Work out the finished part from the listing and answer in its coordinate system (mm). A direction names the side the tool comes from. Coordinates: 2 decimals unless noted, no trailing zeros. Order: outer loops, then holes, each group sorted by start corner. A loop starts at its lowest first (then second) coordinate and runs counter-clockwise, first axis right, second up. Notation, with made-up numbers: (-14.75, 9.5) -> (13.25, 9.5) arc R25 ccw to (13.25, 38.5) -> close; hole circle Ø1 at (70.25, 55.5). An arc over 180 degrees is marked (long way). Use one line per item in the form item = value.
from build123d import *

# Parameters (mm, degrees)
BASE_FLANGE1_DEPTH           = 408.432
SKETCH2_W                    = 2.032
SKETCH2_H                    = 34.036
BOSS_EXTRUDE1_DEPTH          = 25.4
EDGE_FLANGE1_STRIP_W         = 14.478
EDGE_FLANGE1_STRIP_H         = 2.032
EDGE_FLANGE1_STRIP_CUT_DEPTH = 34.036
EDGE_FLANGE1_DEPTH           = 34.036
SKETCH6_R                    = 2.4511
CUT_EXTRUDE1_DEPTH           = 438.764339256
SKETCH7_R                    = 4.3688
CUT_EXTRUDE2_DEPTH           = 438.764339256
SKETCH8_R                    = 2.4511
CUT_EXTRUDE3_DEPTH           = 463.94863897
FILLET1_R                    = 3.175


# Sheet-metal steps are written as plain solids
with BuildPart() as part:
    # Sketch1 → Base-Flange1 (new body)
    with BuildSketch(Plane(origin=(0, 0, 0), x_dir=(0, 0, -1), z_dir=(1, 0, 0))):
        with BuildLine():
            Line((22.225, 0), (5.207, 0))
            ThreePointArc((5.207, 0), (1.52509499, 1.52509499), (0, 5.207))
            Line((0, 5.207), (0, 39.243))
            ThreePointArc((0, 39.243), (1.52509499, 42.92490501), (5.207, 44.45))
            Line((5.207, 44.45), (22.225, 44.45))
            Line((22.225, 44.45), (22.225, 42.418))
            Line((22.225, 42.418), (5.207, 42.418))
            ThreePointArc((5.207, 42.418), (2.96193597, 41.48806403), (2.032, 39.243))
            Line((2.032, 39.243), (2.032, 5.207))
            ThreePointArc((2.032, 5.207), (2.96193597, 2.96193597), (5.207, 2.032))
            Line((5.207, 2.032), (22.225, 2.032))
            Line((22.225, 2.032), (22.225, 0))
        make_face()
    extrude(amount=BASE_FLANGE1_DEPTH)

    # Sketch2 → Boss-Extrude1 (add)
    with BuildSketch(Plane(origin=(408.432, 0, 0), x_dir=(0, 0, -1), z_dir=(1, 0, 0))):
        with Locations((1.016, 22.225)):
            Rectangle(SKETCH2_W, SKETCH2_H)
    boss_extrude1 = extrude(amount=BOSS_EXTRUDE1_DEPTH)

    # Edge-Flange1 strip (across the edge) → Edge-Flange1 strip cut (cut)
    with BuildSketch(Plane(origin=(433.832, 39.243, -2.032), x_dir=(-1, 0, 0), z_dir=(0, -1, 0))):
        with Locations((-2.032, -1.016)):
            Rectangle(EDGE_FLANGE1_STRIP_W, EDGE_FLANGE1_STRIP_H)
    edge_flange1_strip_cut = extrude(amount=EDGE_FLANGE1_STRIP_CUT_DEPTH, mode=Mode.SUBTRACT)

    # Edge-Flange1 section (across the edge) → Edge-Flange1 (add)
    with BuildSketch(Plane(origin=(433.832, 39.243, -2.032), x_dir=(-1, 0, 0), z_dir=(0, -1, 0))):
        with BuildLine():
            Line((0, 3.175), (0, 36.068))
            Line((0, 36.068), (2.032, 36.068))
            Line((2.032, 36.068), (2.032, 3.175))
            ThreePointArc((2.032, 3.175), (2.96193597, 0.92993597), (5.207, 0))
            Line((5.207, 0), (5.207, -2.032))
            ThreePointArc((5.207, -2.032), (1.52509499, -0.50690501), (0, 3.175))
        make_face()
    edge_flange1 = extrude(amount=EDGE_FLANGE1_DEPTH)

    # Mirror1: Boss-Extrude1, Edge-Flange1 strip cut, Edge-Flange1 across plane
    add(boss_extrude1.mirror(Plane.ZY.offset(-204.216)))
    add(edge_flange1_strip_cut.mirror(Plane.ZY.offset(-204.216)), mode=Mode.SUBTRACT)
    add(edge_flange1.mirror(Plane.ZY.offset(-204.216)))

    # Sketch6 → Cut-Extrude1 (cut, through all)
    with BuildSketch(Plane(origin=(0, 44.45, 0), x_dir=(1, 0, 0), z_dir=(0, 1, 0))):
        with Locations(Location((25.4, 15.875, 0), (0, 0, 270))):
            Circle(SKETCH6_R)
        with Locations(Location((383.032, 15.875, 0), (0, 0, 270))):
            Circle(SKETCH6_R)
    extrude(amount=-CUT_EXTRUDE1_DEPTH, mode=Mode.SUBTRACT)

    # Sketch7 → Cut-Extrude2 (cut, through all)
    with BuildSketch(Plane.XY):
        with Locations((50.8, 22.225)):
            Circle(SKETCH7_R)
        with Locations((357.632, 22.225)):
            Circle(SKETCH7_R)
    extrude(amount=-CUT_EXTRUDE2_DEPTH, mode=Mode.SUBTRACT)

    # Sketch8 → Cut-Extrude3 (cut, through all)
    with BuildSketch(Plane(origin=(433.832, 0, 0), x_dir=(0, 0, -1), z_dir=(1, 0, 0))):
        with Locations((31.75, 22.225)):
            Circle(SKETCH8_R)
        with Locations((12.7, 22.225)):
            Circle(SKETCH8_R)
    extrude(amount=-CUT_EXTRUDE3_DEPTH, mode=Mode.SUBTRACT)

    # Fillet1
    fillet1_edges = [part.edges().sort_by_distance(p)[0] for p in [
        (-24.384, 5.207, -38.1),
        (0, 1.016, -22.225),
        (-24.384, 39.243, -38.1),
        (0, 43.434, -22.225),
        (408.432, 1.016, -22.225),
        (432.816, 39.243, -38.1),
        (432.816, 5.207, -38.1),
        (408.432, 43.434, -22.225),
    ]]
    fillet(fillet1_edges, radius=FILLET1_R)


solid = part.part
(1) Section B-B on x = 228 is taken. Write down the section's boundary in (y, z) (3 decimals), plus the area to 3 significant figures.
Data:
outline = (0, -22.225) -> (2.032, -22.225) -> (2.032, -5.207) arc R3.175 cw to (5.207, -2.032) -> (39.243, -2.032) arc R3.175 cw to (42.418, -5.207) -> (42.418, -22.225) -> (44.45, -22.225) -> (44.45, -5.207) arc R5.207 ccw to (39.243, 0) -> (5.207, 0) arc R5.207 ccw to (0, -5.207) -> close
area = 165 mm²
(2) The mould has two halves that part along X. Classify faces 4 (the flat face through (433.832, 22, -21)), 5 (the flat face through (201, 2.032, -14)), 6 (the cylindrical face through (361.8, 23.54, -1)): released by +X, released by -X, zero draft, split by the parting line, or undercut.
Data:
face_4 = released by +X
face_5 = zero draft
face_6 = undercut
(3) Section C-C on y = 31 is taken. Write down the section's boundary in (x, z) (3 decimals), plus the area to 3 significant figures.
Data:
outline = (-25.4, -38.1) -> (-23.368, -38.1) -> (-23.368, -5.207) arc R3.175 cw to (-20.193, -2.032) -> (428.625, -2.032) arc R3.175 cw to (431.8, -5.207) -> (431.8, -38.1) -> (433.832, -38.1) -> (433.832, -5.207) arc R5.207 ccw to (428.625, 0) -> (-20.193, 0) arc R5.207 ccw to (-25.4, -5.207) -> close
area = 1,070 mm²
(4) Section A-A on x = 50.8 is taken. Write down the section's boundary in (y, z) (3 decimals).
Data:
outline = (0, -22.225) -> (2.032, -22.225) -> (2.032, -5.207) arc R3.175 cw to (5.207, -2.032) -> (17.856, -2.032) -> (17.856, 0) -> (5.207, 0) arc R5.207 ccw to (0, -5.207) -> close; (26.594, -2.032) -> (39.243, -2.032) arc R3.175 cw to (42.418, -5.207) -> (42.418, -22.225) -> (44.45, -22.225) -> (44.45, -5.207) arc R5.207 ccw to (39.243, 0) -> (26.594, 0) -> close
(5) Straight lines are drawn through the part: line 1 along X through (y, z) = (12, -35.5); line 2 along Y through (x, z) = (433.4, -31.75); line 3 along X through (y, z) = (23, -2). For each, find the intervals that lie inside material, in ascending order.
Data:
line_1 = -25.4 to -23.37, 431.8 to 433.83
line_2 = 5.21 to 19.77, 24.68 to 39.24
line_3 = -24.3 to 46.5, 55.1 to 353.33, 361.93 to 432.73
(6) Each of these flat-tipped pins is pushed along its axis until it touches: P1, Ø1, axis at x = 302.5, y = 0.5, coming from the -Z side (3 decimals); P2, Ø14, axis at x = 50.8, y = 22.225, coming from the -Z side; P3, Ø5.5, axis at y = 1.5, z = -5, coming from the -X side. Where does it stop, or does it pass through?
Data:
P1 = -22.225
P2 = -2.03
P3 = 0
(7) Which of the six approach directions +Z, -Z, +X, -X, +Y, -Y give full straight-line access (tool end or side, diameter ignored) to faces 1 (the flat face through (432, 39.243, -10)), 2 (the flat face through (207, 22, -2.032)), 3 (the flat face through (201, 42.418, -14))?
Data:
face_1 = +Z, -Z, +X, +Y
face_2 = -Z
face_3 = -Z, +X, -X
